Can you work these out from the model? Positions are in its coordinate system, mm. A direction names the side the tool comes from. Coordinates: 2 decimals unless noted, no trailing zeros. Order: outer loops, then holes, each group sorted by start corner. A loop starts at its lowest first (then second) coordinate and runs counter-clockwise, first axis right, second up. Notation, with made-up numbers: (21, 79) - (71, 79) arc R29 cw to (71, 103) - close; hole circle Ø4 at (27, 16.5). An arc over 180 degrees is marked (long way). Use a Markdown table: item, result. Add a question column.
(1) If I drill on L1, parallel to Y at x = 0, z = 5; L2, parallel to Y at x = 0, z = 7.25; L3, parallel to Y at x = 20, z = 4.25, over which ranges is the centre line in solid material (lowest first)? Write a range as [from, to].
(2) For pin 1 Ø6.5 at (x, y) = (19.05, -11) entering from +Z; pin 2 Ø8 at (x, y) = (-19.05, 11) entering from -Z; pin 3 Ø4 at (x, z) = (-11, 4.5) entering from -Y; pin 4 Ø1 at (y, z) = (-7.5, 6) entering from +X, each with a flat end and sliding along its axis, tell me the tip position at first contact or that it passes through.
(3) I want a section at B-B (z = 1.75). List the corners of the cut face in (x, y) for me.
(4) I want a section at D-D (y = -17). List the corners of the cut face in (x, z) for me, and give its area (3 significant figures).
(5) On a 3-axis mill with a long thin cutter (end or side, diameter ignored), from which of +Z, -Z, +X, -X, +Y, -Y can I reach the whole of each face in a straight line? I mean faces 4 (the cylindrical face through (-21.36, -11.96, 5.73)), 5 (the flat face through (3.2, 3.2, 7)). Say none if no direction works.
(6) I want a section at C-C (x = -25). List the corners of the cut face in (y, z) for me.
(7) I want a section at A-A (y = 0). List the corners of the cut face in (x, z) for me.
(8) We'd pull the mould along X, two halves only. Please class faces 1 (the flat face through (8, 1, 8)), 2 (the cylindrical face through (0.33, -19.52, 5.73)), 3 (the cylindrical face through (21.77, 34.15, 3.94)): pulls with the +X half, pulls with the -X half, needs draft (parallel to the pull), parting line crosses it, or undercut.
```python
from build123d import *

# Parameters (mm, degrees)
F0_R           = 40.5
F1_DEPTH       = 8
F3_D           = 5
F3_CSINK_D     = 6
F3_CSINK_ANGLE = 90
F4_R           = 7.5
F5_DEPTH       = 7
F6_R           = 4.25
F7_DEPTH       = 1.001
F8_W           = 57
F8_H           = 57
F8_R           = 2.5
F8_R_2         = 7.5
F9_DEPTH       = 4
F10_R          = 5


# Not quite as in the source:
# - a feature names something its author has since deleted; it is built from what else it names


with BuildPart() as f1:
    # F0 (on Top) → F1 (new body)
    with BuildSketch(Plane.XY):
        Circle(F0_R)
    extrude(amount=F1_DEPTH)

    # F3 (through all)
    with Locations(Plane.XY.offset(8)):
        with Locations((0, 22), (19.0525588833, 11), (19.0525588833, -11), (0, -22), (-19.0525588833, -11), (-19.0525588833, 11)):
            CounterSinkHole(F3_D / 2, F3_CSINK_D / 2, counter_sink_angle=F3_CSINK_ANGLE)

    # F4 (on face) → F5 (cut)
    with BuildSketch(Plane(origin=(0, 0, 0), x_dir=(1, 0, 0), z_dir=(0, 0, -1))):
        Circle(F4_R)
    extrude(amount=-F5_DEPTH, mode=Mode.SUBTRACT)

    # F6 (on face) → F7 (cut, through all)
    with BuildSketch(Plane(origin=(0, 0, 7), x_dir=(1, 0, 0), z_dir=(0, 0, -1))):
        Circle(F6_R)
    extrude(amount=-F7_DEPTH, mode=Mode.SUBTRACT)

    # F8 (on face) → F9 (cut)
    with BuildSketch(Plane(origin=(0, 0, 0), x_dir=(1, 0, 0), z_dir=(0, 0, -1))):
        Rectangle(F8_W, F8_H)
        with Locations((-19.0525588833, -11)):
            Circle(F8_R, mode=Mode.SUBTRACT)
        with Locations((0, -22)):
            Circle(F8_R, mode=Mode.SUBTRACT)
        with Locations((19.0525588833, -11)):
            Circle(F8_R, mode=Mode.SUBTRACT)
        with Locations((-19.0525588833, 11)):
            Circle(F8_R, mode=Mode.SUBTRACT)
        Circle(F8_R_2, mode=Mode.SUBTRACT)
        with Locations((19.0525588833, 11)):
            Circle(F8_R, mode=Mode.SUBTRACT)
        with Locations((0, 22)):
            Circle(F8_R, mode=Mode.SUBTRACT)
    extrude(amount=-F9_DEPTH, mode=Mode.SUBTRACT)

    # F10
    f10_edges = [f1.edges().sort_by_distance(p)[0] for p in [
        (28.5, 28.5, 2),
        (28.5, -28.5, 2),
        (-28.5, -28.5, 2),
        (-28.5, 28.5, 2),
    ]]
    fillet(f10_edges, radius=F10_R)


solid = f1.part
```
Answers follow:
| question | item | result |
|---|---|---|
| 1 | L1 | y = [-40.5, -24.5], [-19.5, -7.5], [7.5, 19.5], [24.5, 40.5] |
| 1 | L2 | y = [-40.5, -24.5], [-19.5, -4.25], [4.25, 19.5], [24.5, 40.5] |
| 1 | L3 | y = [-35.22, -13.31], [-8.69, 8.69], [13.31, 35.22] |
| 2 | pin 1 | stops at z = 8 |
| 2 | pin 2 | stops at z = 4 |
| 2 | pin 3 | stops at y = -39.49 |
| 2 | pin 4 | stops at x = 39.89 |
| 3 | outline | circle Ø81 at (0, 0); hole (-28.5, -23.5) arc R5 ccw to (-23.5, -28.5) - (23.5, -28.5) arc R5 ccw to (28.5, -23.5) - (28.5, 23.5) arc R5 ccw to (23.5, 28.5) - (-23.5, 28.5) arc R5 ccw to (-28.5, 23.5) - close |
| 4 | outline | (-36.76, 0) - (-28.5, 0) - (-28.5, 4) - (28.5, 4) - (28.5, 0) - (36.76, 0) - (36.76, 8) - (-36.76, 8) - close |
| 4 | area | 360 mm² |
| 5 | face 4 | +Z, -Z |
| 5 | face 5 | -Z |
| 6 | outline | (-31.86, 0) - (-28.27, 0) - (-28.27, 4) - (28.27, 4) - (28.27, 0) - (31.86, 0) - (31.86, 8) - (-31.86, 8) - close |
| 7 | outline | (-40.5, 0) - (-28.5, 0) - (-28.5, 4) - (-7.5, 4) - (-7.5, 7) - (-4.25, 7) - (-4.25, 8) - (-40.5, 8) - close; (4.25, 7) - (7.5, 7) - (7.5, 4) - (28.5, 4) - (28.5, 0) - (40.5, 0) - (40.5, 8) - (4.25, 8) - close |
| 8 | face 1 | needs draft |
| 8 | face 2 | undercut |
| 8 | face 3 | parting line crosses it |
